```python
from build123d import *

# Parameters (mm, degrees)
SKETCH2_W           = 160
SKETCH2_H           = 60
BOSS_EXTRUDE1_DEPTH = 230
CUT_EXTRUDE1_REACH  = 162
SHELL1_T            = -10
SKETCH5_R           = 5
CUT_EXTRUDE2_DEPTH  = 161


with BuildPart() as part:
    # Sketch2 → Boss-Extrude1 (new body)
    with BuildSketch(Plane.XY):
        Rectangle(SKETCH2_W, SKETCH2_H)
    extrude(amount=BOSS_EXTRUDE1_DEPTH)

    # Sketch3 → Cut-Extrude1 (cut, up to next)
    with BuildSketch(Plane(origin=(80, 0, 0), x_dir=(0, 0, -1), z_dir=(1, 0, 0)), mode=Mode.PRIVATE) as cut_extrude1_sk1:
        Polygon((-100, 30), (-203.923048454, -30), (-230, -30), (-230, 30), align=None)
    cut_extrude1_tool1 = extrude(cut_extrude1_sk1.sketch, amount=-CUT_EXTRUDE1_REACH, mode=Mode.PRIVATE) & part.part
    add(cut_extrude1_tool1.solids().sort_by_distance((80, 6.658449, 185.214376))[0], mode=Mode.SUBTRACT)

    # Shell1
    shell1_openings = [part.faces().sort_by_distance(p)[0] for p in [
        (0, -30, 101.961524227),
    ]]
    offset(amount=SHELL1_T, openings=shell1_openings, kind=Kind.INTERSECTION)

    # Sketch5 → Cut-Extrude2 (cut, through all)
    with BuildSketch(Plane(origin=(80, 0, 0), x_dir=(0, 0, -1), z_dir=(1, 0, 0))):
        with Locations((-23, 0)):
            Circle(SKETCH5_R)
    extrude(amount=-CUT_EXTRUDE2_DEPTH, mode=Mode.SUBTRACT)


solid = part.part
```
Read the model definition and answer for the solid it produces. Units are mm, in the model's axes. A direction names the side the tool comes from. Coordinates: 2 decimals unless noted, no trailing zeros. Write each loop counter-clockwise with the first axis right and the second up, starting at its lowest first coordinate (ties: lowest second). Pieces come first, ordered by that corner, then holes. Notation, with made-up numbers: (8.5, 80) -> (37.5, 80) arc R21 ccw to (37.5, 88) -> close; hole circle Ø3 at (56, -5.5). An arc over 180 degrees is marked (long way). Answer as a JSON object with one key per item and string values.
Q1. The part is cut by section B-B on y = -8.5. Give the vertices of the cut face in (x, z), then the cut area to 3 significant figures.
The answers:
{"outline": "(-80, 0) -> (80, 0) -> (80, 166.68) -> (-80, 166.68) -> close; hole (-70, 10) -> (70, 10) -> (70, 146.68) -> (-70, 146.68) -> close", "area": "7,530 mm2"}
Q2. The part is cut by section A-A on z = 23. Give the vertices of the cut face in (x, y).
The answers:
{"outline": "(-80, -30) -> (-70, -30) -> (-70, -5) -> (-80, -5) -> close; (-80, 5) -> (-70, 5) -> (-70, 20) -> (70, 20) -> (70, 5) -> (80, 5) -> (80, 30) -> (-80, 30) -> close; (70, -30) -> (80, -30) -> (80, -5) -> (70, -5) -> close"}
Q3. The part is cut by section D-D on z = 122. Give the vertices of the cut face in (x, y).
The answers:
{"outline": "(-80, -30) -> (-70, -30) -> (-70, 5.75) -> (70, 5.75) -> (70, -30) -> (80, -30) -> (80, 17.3) -> (-80, 17.3) -> close"}
Q4. The part is cut by section C-C on x = 9.5. Give the vertices of the cut face in (y, z).
The answers:
{"outline": "(-30, 0) -> (30, 0) -> (30, 100) -> (-30, 203.92) -> (-30, 183.92) -> (20, 97.32) -> (20, 10) -> (-30, 10) -> close"}
Q5. Consider line 1 (X direction, y = -23.5, z = 39.5); line 2 (Y direction, x = 75, z = 23); line 3 (Y direction, x = 58.5, z = 67). Determine where each line is inside the solid, lowest interval first. Write a range as [from, to].
The answers:
{"line 1": "x = [-80, -70], [70, 80]", "line 2": "y = [-30, -5], [5, 30]", "line 3": "y = [20, 30]"}
Q6. A tool of negligible diameter and unlimited length cuts with its end or side. For faces 1 (the cylindrical face through (-75, 0, 28)), 2 (the flat face through (-1, 20, 53)), from which of +Z, -Z, +X, -X, +Y, -Y can it reach the whole face along a straight path? Write none if from no direction.
The answers:
{"face 1": "+X, -X", "face 2": "-Y"}
Q7. Determine the mould class of faces 3 (the flat face through (-1, 30, 49)), 4 (the cylindrical face through (75, 0, 28)), 5 (the flat face through (-1, 0, 0)) for opening direction Z: pulls with the +Z half, pulls with the -Z half, needs draft (parallel to the pull), parting line crosses it, or undercut.
The answers:
{"face 3": "needs draft", "face 4": "undercut", "face 5": "pulls with the -Z half"}
Q8. Flat-ended cylindrical pins translate along their axes: pin 1 Ø1.5 at (x, y) = (32.5, 1.5) entering from +Z; pin 2 Ø5 at (x, y) = (-38, 20) entering from +Z; pin 3 Ø12 at (x, y) = (27.5, -7) entering from +Z. Find the tip coordinate at first contact, or state that the pin passes through.
The answers:
{"pin 1": "stops at z = 150.66", "pin 2": "stops at z = 121.65", "pin 3": "stops at z = 174.48"}
